Input: part model. Units: mm. Frame: model coordinates. A direction names the side the tool comes from. Coordinates: 2 decimals unless noted, no trailing zeros. Write each loop counter-clockwise with the first axis right and the second up, starting at its lowest first coordinate (ties: lowest second). Pieces come first, ordered by that corner, then holes. Notation, with made-up numbers: (76, 42) - (127, 42) arc R7 ccw to (127, 55) - close; hole circle Ø7 at (42.5, 81.25). An arc over 180 degrees is marked (long way). Use a Markdown table: item, result. Add a question column.
Q1. Set-up query: faces 1 (the face through (45, 0, -279)), 2 (the face through (0.22, 42.49, -260.91)), 3 (the face through (-45, 0, -279)). Return all of +Z, -Z, +X, -X, +Y, -Y with unobstructed straight access to the full face (end or side cutting, diameter ignored); none if empty.
Q2. Section query C-C (x = -1). Return the cut outline in (y, z) (3 decimals), then the cut area to 3 significant figures.
Q3. Section query D-D (y = 249). Return the cut outline in (x, z) (3 decimals).
Q4. Section query A-A (x = 38.1). Return the cut outline in (y, z) (3 decimals), then the cut area to 3 significant figures.
Q5. Material intervals for probe 1 along X at (y, z) = (-6, -279); probe 2 along Y at (x, z) = (10.5, -88.5); probe 3 along X at (y, z) = (48, -133.5) (3 decimals), sorted ascending. Write a range as from..to.
Q6. Section query B-B (z = 279.4). Return the cut outline in (x, y) (3 decimals).
Q7. Mould query, pull axis Y, two halves, no side actions, for faces 4 (the face through (-45, 0, 280)), 5 (the face through (0.222, 269.625, -186.967)), 6 (the face through (-32.466, -5.009, -276.47)), 7 (the face through (0, 0, 4)). Classes: released by +Y, released by -Y, zero draft, split by the parting line, or undercut.
Q8. Pin query (flat end, axial travel): P1, Ø16, axis at x = -42, z = -280, coming from the +Y side; P2, Ø10, axis at x = -8.5, z = 96.5, coming from the -Y side; P3, Ø7.5, axis at x = 38.1, z = -279.4, coming from the -Y side; P4, Ø12, axis at x = -21.5, y = 112.5, coming from the +Z side. Return the tip coordinate at first contact, or that it passes through.
from build123d import *

# Parameters (mm, degrees)
BOSS_EXTRUDE1_DEPTH = 15.875
FILLET1_R           = 38.1
FILLET2_R           = 50.8
SKETCH2_W           = 127
SKETCH2_H           = 31.75
SKETCH2_R           = 6.35
BOSS_EXTRUDE2_DEPTH = 10.16
FILLET3_R           = 2.54


with BuildPart() as part:
    # Sketch1 → Boss-Extrude1 (new, symmetric)
    with BuildSketch(Plane(origin=(0, 0, 0), x_dir=(0, 0, -1), z_dir=(1, 0, 0))):
        with BuildLine():
            Line((-304.8, 0), (304.8, 0))
            Line((304.8, 0), (304.8, 38.1))
            Line((304.8, 38.1), (177.8, 50.8))
            ThreePointArc((177.8, 50.8), (182.64153721, 255.463845718), (286.642935854, 431.8))
            Line((286.642935854, 431.8), (261.242935854, 431.8))
            ThreePointArc((261.242935854, 431.8), (141.525824012, 273.647129076), (110.92514038, 77.667243347))
            ThreePointArc((110.92514038, 77.667243347), (104.653146696, 58.510068346), (86.40105547, 49.954577438))
            Line((86.40105547, 49.954577438), (-304.8, 38.1))
            Line((-304.8, 38.1), (-304.8, 0))
        make_face()
    extrude(amount=BOSS_EXTRUDE1_DEPTH, both=True)

    # Fillet1
    fillet1_edges = [part.edges().sort_by_distance(p)[0] for p in [
        (0, 431.8, -261.242935854),
    ]]
    fillet(fillet1_edges, radius=FILLET1_R)

    # Fillet2
    fillet2_edges = [part.edges().sort_by_distance(p)[0] for p in [
        (0, 50.8, -177.8),
    ]]
    fillet(fillet2_edges, radius=FILLET2_R)

    # Sketch2 → Boss-Extrude2 (add)
    # profile 1 of 2: a face of its own
    with BuildSketch(Plane.XZ):
        with Locations((0, 279.4)):
            Rectangle(SKETCH2_W, SKETCH2_H)
        with Locations(Location((-38.1, 279.4, 0), (0, 0, 270))):
            Circle(SKETCH2_R, mode=Mode.SUBTRACT)
        with Locations(Location((38.1, 279.4, 0), (0, 0, 270))):
            Circle(SKETCH2_R, mode=Mode.SUBTRACT)
    # profile 2 of 2: a face of its own
    with BuildSketch(Plane.XZ):
        with Locations((0, -279.4)):
            Rectangle(SKETCH2_W, SKETCH2_H)
        with Locations(Location((38.1, -279.4, 0), (0, 0, 90))):
            Circle(SKETCH2_R, mode=Mode.SUBTRACT)
        with Locations(Location((-38.1, -279.4, 0), (0, 0, 90))):
            Circle(SKETCH2_R, mode=Mode.SUBTRACT)
    extrude(amount=BOSS_EXTRUDE2_DEPTH)

    # Fillet3
    fillet3_edges = [part.edges().sort_by_distance(p)[0] for p in [
        (0, 431.8, -286.642935854),
    ]]
    fillet(fillet3_edges, radius=FILLET3_R)


solid = part.part
Values follow:
| question | item | result |
|---|---|---|
| 1 | face 1 | +Z, -Z, +X, +Y |
| 1 | face 2 | -Z, +X, -X |
| 1 | face 3 | +Z, -Z, -X, +Y |
| 2 | outline | (-10.16, -295.275) - (0, -295.275) - (0, -304.8) - (38.1, -304.8) - (47.002, -215.778) arc R50.8 cw to (90.939, -170.465) arc R406.4 cw to (427.487, -282.376) arc R2.54 ccw to (431.8, -280.557) - (431.8, -275.014) arc R38.1 ccw to (422.546, -250.124) arc R406.4 ccw to (77.667, -110.925) arc R25.4 cw to (49.955, -86.401) - (38.1, 304.8) - (0, 304.8) - (0, 295.275) - (-10.16, 295.275) - (-10.16, 263.525) - (0, 263.525) - (0, -263.525) - (-10.16, -263.525) - close |
| 2 | area | 46,900 mm2 |
| 3 | outline | (-15.875, -180.853) - (15.875, -180.853) - (15.875, -131.997) - (-15.875, -131.997) - close |
| 4 | outline | (-10.16, -295.275) - (0, -295.275) - (0, -285.75) - (-10.16, -285.75) - close; (-10.16, -273.05) - (0, -273.05) - (0, -263.525) - (-10.16, -263.525) - close; (-10.16, 263.525) - (0, 263.525) - (0, 273.05) - (-10.16, 273.05) - close; (-10.16, 285.75) - (0, 285.75) - (0, 295.275) - (-10.16, 295.275) - close |
| 4 | area | 387 mm2 |
| 5 | probe 1 | -63.5..-44.44, -31.76..31.76, 44.44..63.5 |
| 5 | probe 2 | 0..50.11 |
| 5 | probe 3 | -15.875..15.875 |
| 6 | outline | (-63.5, -10.16) - (-44.45, -10.16) - (-44.45, 0) - (-63.5, 0) - close; (-31.75, -10.16) - (31.75, -10.16) - (31.75, 0) - (15.875, 0) - (15.875, 38.87) - (-15.875, 38.87) - (-15.875, 0) - (-31.75, 0) - close; (44.45, -10.16) - (63.5, -10.16) - (63.5, 0) - (44.45, 0) - close |
| 7 | face 4 | released by +Y |
| 7 | face 5 | undercut |
| 7 | face 6 | zero draft |
| 7 | face 7 | released by -Y |
| 8 | P1 | y = 0 |
| 8 | P2 | y = 0 |
| 8 | P3 | through |
| 8 | P4 | z = -109.22 |
